from build123d import *

# Parameters (mm, degrees)
EXTRUDE_1_DEPTH     = 17.5
EXTRUDE_2_DEPTH     = 3
EXTRUDE_START       = 5
SKETCH_5_R          = 6
SKETCH_5_R_2        = 3
EXTRUDE_3_DEPTH     = 10
SKETCH_2_R          = 3
CUT_EXTRUDE_1_DEPTH = 6


with BuildPart() as part:
    # 草圖1 → 填料-伸長1 (new body, symmetric)
    with BuildSketch(Plane.XY):
        Polygon((-7, 0), (7, 0), (7, -5), (5, -5), (5, -3), (-5, -3), (-5, -5), (-7, -5), align=None)
    extrude(amount=EXTRUDE_1_DEPTH, both=True)

    # 草圖4 → 填料-伸長2 (add, symmetric)
    with BuildSketch(Plane.XY):
        Polygon((-7, 0), (20, 15), (25, 15), (25, 5), (7, -5), (7, 0), align=None)
    extrude(amount=EXTRUDE_2_DEPTH, both=True)

    # 草圖5 → 填料-伸長3 (add)
    with BuildSketch(Plane(origin=(0, 0, 0), x_dir=(1, 0, 0), z_dir=(0, 1, 0)).offset(EXTRUDE_START)):
        with Locations((30, 0)):
            Circle(SKETCH_5_R)
        with Locations((30, 0)):
            Circle(SKETCH_5_R_2, mode=Mode.SUBTRACT)
    extrude(amount=EXTRUDE_3_DEPTH)

    # 草圖2 → 除料-伸長1 (cut, through all)
    with BuildSketch(Plane(origin=(0, 0, 0), x_dir=(1, 0, 0), z_dir=(0, 1, 0))):
        with Locations((0, -10)):
            Circle(SKETCH_2_R)
        with Locations((0, 10)):
            Circle(SKETCH_2_R)
    extrude(amount=-CUT_EXTRUDE_1_DEPTH, mode=Mode.SUBTRACT)


solid = part.part
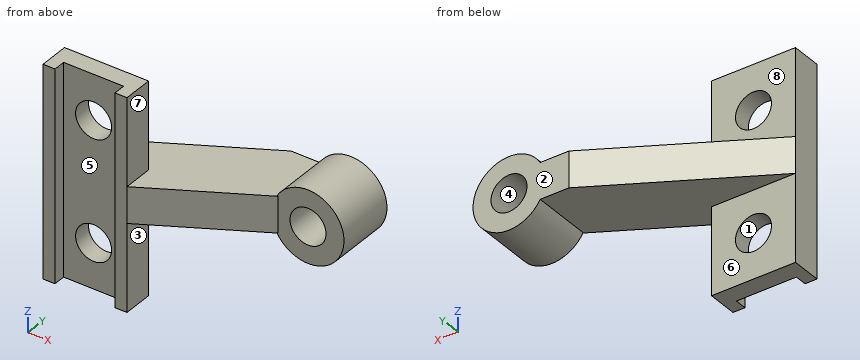
Part model, mm, in its own coordinate system. Face numbers are marked on the shaded views. A direction names the side the tool comes from. Coordinates: 2 decimals unless noted, no trailing zeros. Loops run counter-clockwise (first coordinate to the right, second up) from the corner with the lowest first, then second, coordinate; pieces in that order, holes last. Notation, with made-up numbers: (-10.75, -9.5) -> (29.25, -9.5) arc R7 cw to (29.25, 2.5) -> close; hole circle Ø2 at (36.5, 70.25). An arc over 180 degrees is marked (long way). Use a Markdown table: item, result. Add a question column.
Item 1: Pull direction X, two halves, no side cores. Call the marked faces 1, 2, 3 and 4: +X half, -X half, draft (parallel to the pull), parting line (faces both ways), or undercut.
Item 2: Band-saw the part on D-D on z = -13.5. Write the cut outline in (x, y).
Item 3: Probe probe 1 along Z at (x, y) = (0, -1.1); probe 2 along Z at (x, y) = (30, 8.25); probe 3 along X at (y, z) = (-0.6, 10). List the from-to ranges inside material, lowest first.
Item 4: Flat gauge pins, fed straight in: P1, Ø3, axis at x = 8, y = 3.5, coming from the +Z side; P2, Ø8, axis at y = 4.5, z = -12, coming from the -X side; P3, Ø1.5, axis at y = -2, z = 13, coming from the +X side; P4, Ø11, axis at x = -1, z = 10.5, coming from the +Y side. Where does each tip first touch, or does it go through?
Item 5: Band-saw the part on C-C on y = -1.5. Write the cut outline in (x, z), plus the area to 3 significant figures.
Item 6: Which spindle directions (+Z, -Z, +X, -X, +Y, -Y) get a long thin tool onto all of the face, cutting with end or side? Do the marked faces 5, 6, 7 and 8. Say none if no direction does.
Item 7: Band-saw the part on A-A on z = 0. Write the cut outline in (x, y).
Item 8: Band-saw the part on B-B on x = 30. Write the cut outline in (y, z).
Geometry says:
| question | item | result |
|---|---|---|
| 1 | face 1 | undercut |
| 1 | face 2 | draft |
| 1 | face 3 | +X half |
| 1 | face 4 | undercut |
| 2 | outline | (-7, -5) -> (-5, -5) -> (-5, -3) -> (5, -3) -> (5, -5) -> (7, -5) -> (7, 0) -> (-7, 0) -> close |
| 3 | probe 1 | -17.5 to -13, -7 to 7, 13 to 17.5 |
| 3 | probe 2 | -6 to -3, 3 to 6 |
| 3 | probe 3 | -7 to -3, 3 to 7 |
| 4 | P1 | z = 3 |
| 4 | P2 | through |
| 4 | P3 | x = 7 |
| 4 | P4 | y = 0 |
| 5 | outline | (-7, -17.5) -> (7, -17.5) -> (7, -3) -> (13.3, -3) -> (13.3, 3) -> (7, 3) -> (7, 17.5) -> (-7, 17.5) -> close; hole circle Ø6 at (0, -10); hole circle Ø6 at (0, 10) |
| 5 | area | 471 mm² |
| 6 | face 5 | +Z, -Z, -Y |
| 6 | face 6 | -Z, +X, -X, +Y |
| 6 | face 7 | +Z, +X, +Y, -Y |
| 6 | face 8 | +Z, +X, -X, +Y |
| 7 | outline | (-7, -5) -> (-5, -5) -> (-5, -3) -> (5, -3) -> (5, -5) -> (7, -5) -> (25, 5) -> (27, 5) -> (27, 15) -> (20, 15) -> (-7, 0) -> close; (33, 5) -> (36, 5) -> (36, 15) -> (33, 15) -> close |
| 8 | outline | (5, -6) -> (15, -6) -> (15, -3) -> (5, -3) -> close; (5, 3) -> (15, 3) -> (15, 6) -> (5, 6) -> close |
